Geometry check sheet. Reference: the model listing, model coordinates, mm. Give positions to 0.01 mm unless a question says otherwise; leave off trailing zeros. Write item = value, one per line. Start each with the question number.
1. Depth check by flat-ended pin: P1, Ø4, axis at x = 111.9, z = -118.65, coming from the -Y side. Enter the tip coordinate at first touch or a pass-through.
2. Thickness scan on line 1 along Z through (x, y) = (194.45, 2.4); line 2 along X through (y, z) = (0.55, -153); line 3 along X through (y, z) = (3.5, -16). Record the ranges inside material, lowest first.
3. Mould release check, pull along X, two halves, no side actions. Record for faces 1 (the flat face through (148, 3, 0)), 2 (the flat face through (300, 3, -99)), 3 (the cylindrical face through (146.173, 3.042, -119.501)): pulls with the +X half, pulls with the -X half, needs draft (parallel to the pull), parting line crosses it, or undercut.
```python
from build123d import *

# Parameters (mm, degrees)
SKETCH1_W           = 300
SKETCH1_H           = 200
BOSS_EXTRUDE1_DEPTH = 6
SKETCH6_R           = 4
CUT_EXTRUDE2_DEPTH  = 361.605047108
FILLET1_R           = 6.35
SKETCH2_R           = 1.5
CUT_EXTRUDE1_DEPTH  = 361.605047108
SKETCH13_R          = 1.6
M3_THROUGH2_DEPTH   = 364.853871767
SKETCH16_R          = 2.65
M5_THROUGH_DEPTH    = 358.420816406
SKETCH9_R           = 1.5
CUT_EXTRUDE3_DEPTH  = 361.605047108
SKETCH10_R          = 1.5
CUT_EXTRUDE5_DEPTH  = 361.605047108
SKETCH17_R          = 1.6
M3_THROUGH_DEPTH    = 361.605047108
MOVE_FACE2_BY       = 0.08
MOVE_FACE2_2_BY     = 0.08
MOVE_FACE2_3_BY     = 0.08
MOVE_FACE2_4_BY     = 0.08
MOVE_FACE2_5_BY     = 0.08
MOVE_FACE2_6_BY     = 0.08
MOVE_FACE2_7_BY     = 0.08
MOVE_FACE2_8_BY     = 0.08
MOVE_FACE2_9_BY     = 0.08
MOVE_FACE2_10_BY    = 0.08
MOVE_FACE2_11_BY    = 0.08
MOVE_FACE2_12_BY    = 0.08
MOVE_FACE2_13_BY    = 0.08
MOVE_FACE2_14_BY    = 0.08
MOVE_FACE2_15_BY    = 0.08
MOVE_FACE2_16_BY    = 0.08
MOVE_FACE2_17_BY    = 0.08
MOVE_FACE2_18_BY    = 0.08
MOVE_FACE2_19_BY    = 0.08
MOVE_FACE2_20_BY    = 0.08
MOVE_FACE2_21_BY    = 0.08
MOVE_FACE2_22_BY    = 0.08
MOVE_FACE2_23_BY    = 0.08
MOVE_FACE2_24_BY    = 0.08
MOVE_FACE2_25_BY    = 0.08
MOVE_FACE2_26_BY    = 0.08
MOVE_FACE2_27_BY    = 0.08
MOVE_FACE2_28_BY    = 0.08
MOVE_FACE2_29_BY    = 0.08
MOVE_FACE2_30_BY    = 0.08
MOVE_FACE2_31_BY    = 0.08
MOVE_FACE2_32_BY    = 0.08
MOVE_FACE2_33_BY    = 0.08
MOVE_FACE2_34_BY    = 0.08
MOVE_FACE2_35_BY    = 0.08
MOVE_FACE2_36_BY    = 0.08
MOVE_FACE2_37_BY    = 0.08
MOVE_FACE2_38_BY    = 0.08
MOVE_FACE2_39_BY    = 0.08
MOVE_FACE2_40_BY    = 0.08


with BuildPart() as part:
    # Sketch1 → Boss-Extrude1 (new body)
    with BuildSketch(Plane(origin=(0, 0, 0), x_dir=(1, 0, 0), z_dir=(0, 1, 0))):
        with Locations((150, 100)):
            Rectangle(SKETCH1_W, SKETCH1_H)
    extrude(amount=BOSS_EXTRUDE1_DEPTH)

    # Sketch6 → Cut-Extrude2 (cut, through all)
    with BuildSketch(Plane(origin=(0, 6, 0), x_dir=(1, 0, 0), z_dir=(0, 1, 0))):
        with Locations(Location((150, 118.65102, 0), (0, 0, 270))):
            Circle(SKETCH6_R)
    extrude(amount=-CUT_EXTRUDE2_DEPTH, mode=Mode.SUBTRACT)

    # Fillet1
    fillet1_edges = [part.edges().sort_by_distance(p)[0] for p in [
        (0, 3, -200),
        (300, 3, -200),
        (300, 3, 0),
        (0, 3, 0),
    ]]
    fillet(fillet1_edges, radius=FILLET1_R)

    # Sketch2 → Cut-Extrude1 (cut, through all)
    with BuildSketch(Plane(origin=(0, 6, 0), x_dir=(1, 0, 0), z_dir=(0, 1, 0))):
        with Locations(Location((6.35, 174.6, 0), (0, 0, 270))):
            Circle(SKETCH2_R)
        with Locations(Location((6.35, 49.9999, 0), (0, 0, 270))):
            Circle(SKETCH2_R)
        with Locations(Location((293.65, 49.9999, 0), (0, 0, 270))):
            Circle(SKETCH2_R)
        with Locations(Location((293.65, 174.6, 0), (0, 0, 270))):
            Circle(SKETCH2_R)
    extrude(amount=-CUT_EXTRUDE1_DEPTH, mode=Mode.SUBTRACT)

    # Sketch13 → M3-through2 (cut, through all)
    with BuildSketch(Plane(origin=(0, 6, 5.8), x_dir=(1, 0, 0), z_dir=(0, 1, 0))):
        with Locations(Location((6.35, 199.45, 0), (0, 0, 270))):
            Circle(SKETCH13_R)
        with Locations(Location((78.175, 199.45, 0), (0, 0, 270))):
            Circle(SKETCH13_R)
        with Locations(Location((221.825, 199.45, 0), (0, 0, 270))):
            Circle(SKETCH13_R)
        with Locations(Location((293.65, 199.45, 0), (0, 0, 270))):
            Circle(SKETCH13_R)
        with Locations(Location((293.65, 99.4498, 0), (0, 0, 270))):
            Circle(SKETCH13_R)
        with Locations(Location((293.65, 12.15, 0), (0, 0, 270))):
            Circle(SKETCH13_R)
        with Locations(Location((217.45, 12.15, 0), (0, 0, 270))):
            Circle(SKETCH13_R)
        with Locations(Location((82.55, 12.15, 0), (0, 0, 270))):
            Circle(SKETCH13_R)
        with Locations(Location((6.35, 12.15, 0), (0, 0, 270))):
            Circle(SKETCH13_R)
        with Locations(Location((6.35, 99.4498, 0), (0, 0, 270))):
            Circle(SKETCH13_R)
    extrude(amount=-M3_THROUGH2_DEPTH, mode=Mode.SUBTRACT)

    # Sketch16 → M5_through (cut, through all)
    with BuildSketch(Plane(origin=(0, 6, -5.8), x_dir=(1, 0, 0), z_dir=(0, -1, 0))):
        with Locations(Location((118.25, -18.65102, 0), (0, 0, 270))):
            Circle(SKETCH16_R)
        with Locations(Location((118.25, -0.55098, 0), (0, 0, 270))):
            Circle(SKETCH16_R)
        with Locations(Location((139.416666667, -0.55098, 0), (0, 0, 270))):
            Circle(SKETCH16_R)
        with Locations(Location((160.583333333, -0.55098, 0), (0, 0, 270))):
            Circle(SKETCH16_R)
        with Locations(Location((181.75, -0.55098, 0), (0, 0, 270))):
            Circle(SKETCH16_R)
        with Locations(Location((181.75, -18.65102, 0), (0, 0, 270))):
            Circle(SKETCH16_R)
    extrude(amount=M5_THROUGH_DEPTH, mode=Mode.SUBTRACT)

    # Sketch9 → Cut-Extrude3 (cut, through all)
    with BuildSketch(Plane(origin=(0, 6, 0), x_dir=(-1, 0, 0), z_dir=(0, 1, 0))):
        with Locations(Location((-118.25, -15.401, 0), (0, 0, 90))):
            Circle(SKETCH9_R)
        with Locations(Location((-150, -6.35098, 0), (0, 0, 90))):
            Circle(SKETCH9_R)
        with Locations(Location((-181.75, -15.401, 0), (0, 0, 90))):
            Circle(SKETCH9_R)
    extrude(amount=-CUT_EXTRUDE3_DEPTH, mode=Mode.SUBTRACT)

    # Sketch10 → Cut-Extrude5 (cut, through all)
    with BuildSketch(Plane(origin=(0, 6, 0), x_dir=(1, 0, 0), z_dir=(0, 1, 0))):
        with Locations(Location((150, 156.75102, 0), (0, 0, 270))):
            Circle(SKETCH10_R)
        with Locations(Location((182.995567884, 137.70102, 0), (0, 0, 270))):
            Circle(SKETCH10_R)
        with Locations(Location((182.995567884, 99.60102, 0), (0, 0, 270))):
            Circle(SKETCH10_R)
        with Locations(Location((150, 80.55102, 0), (0, 0, 270))):
            Circle(SKETCH10_R)
        with Locations(Location((117.004432116, 99.60102, 0), (0, 0, 270))):
            Circle(SKETCH10_R)
        with Locations(Location((117.004432116, 137.70102, 0), (0, 0, 270))):
            Circle(SKETCH10_R)
        with Locations(Location((105.55, 30.80102, 0), (0, 0, 270))):
            Circle(SKETCH10_R)
        with Locations(Location((105.55, 6.35, 0), (0, 0, 270))):
            Circle(SKETCH10_R)
        with Locations(Location((194.45, 6.35, 0), (0, 0, 90))):
            Circle(SKETCH10_R)
        with Locations(Location((194.45, 30.80102, 0), (0, 0, 90))):
            Circle(SKETCH10_R)
    extrude(amount=-CUT_EXTRUDE5_DEPTH, mode=Mode.SUBTRACT)

    # Sketch17 → M3-through (cut, through all)
    with BuildSketch(Plane(origin=(0, 6, 0), x_dir=(1, 0, 0), z_dir=(0, 1, 0))):
        with Locations(Location((188.1, 118.65102, 0), (0, 0, 270))):
            Circle(SKETCH17_R)
        with Locations(Location((169.05, 85.655452116, 0), (0, 0, 270))):
            Circle(SKETCH17_R)
        with Locations(Location((130.95, 85.655452116, 0), (0, 0, 270))):
            Circle(SKETCH17_R)
        with Locations(Location((111.9, 118.65102, 0), (0, 0, 270))):
            Circle(SKETCH17_R)
        with Locations(Location((130.95, 151.646587884, 0), (0, 0, 270))):
            Circle(SKETCH17_R)
        with Locations(Location((169.05, 151.646587884, 0), (0, 0, 270))):
            Circle(SKETCH17_R)
    extrude(amount=-M3_THROUGH_DEPTH, mode=Mode.SUBTRACT)

    # Move Face2: a curved face moved outward by 0.08
    add(Solid.thicken(part.faces().sort_by_distance((150, 3, -122.65102))[0], MOVE_FACE2_BY))

    # Move Face2 2: a curved face moved outward by 0.08
    add(Solid.thicken(part.faces().sort_by_distance((6.35, 3, -176.1))[0], MOVE_FACE2_2_BY))

    # Move Face2 3: a curved face moved outward by 0.08
    add(Solid.thicken(part.faces().sort_by_distance((6.35, 3, -51.4999))[0], MOVE_FACE2_3_BY))

    # Move Face2 4: a curved face moved outward by 0.08
    add(Solid.thicken(part.faces().sort_by_distance((293.65, 3, -51.4999))[0], MOVE_FACE2_4_BY))

    # Move Face2 5: a curved face moved outward by 0.08
    add(Solid.thicken(part.faces().sort_by_distance((293.65, 3, -176.1))[0], MOVE_FACE2_5_BY))

    # Move Face2 6: a curved face moved outward by 0.08
    add(Solid.thicken(part.faces().sort_by_distance((6.35, 3, -195.25))[0], MOVE_FACE2_6_BY))

    # Move Face2 7: a curved face moved outward by 0.08
    add(Solid.thicken(part.faces().sort_by_distance((78.175, 3, -195.25))[0], MOVE_FACE2_7_BY))

    # Move Face2 8: a curved face moved outward by 0.08
    add(Solid.thicken(part.faces().sort_by_distance((221.825, 3, -195.25))[0], MOVE_FACE2_8_BY))

    # Move Face2 9: a curved face moved outward by 0.08
    add(Solid.thicken(part.faces().sort_by_distance((293.65, 3, -195.25))[0], MOVE_FACE2_9_BY))

    # Move Face2 10: a curved face moved outward by 0.08
    add(Solid.thicken(part.faces().sort_by_distance((293.65, 3, -95.2498))[0], MOVE_FACE2_10_BY))

    # Move Face2 11: a curved face moved outward by 0.08
    add(Solid.thicken(part.faces().sort_by_distance((293.65, 3, -7.95))[0], MOVE_FACE2_11_BY))

    # Move Face2 12: a curved face moved outward by 0.08
    add(Solid.thicken(part.faces().sort_by_distance((217.45, 3, -7.95))[0], MOVE_FACE2_12_BY))

    # Move Face2 13: a curved face moved outward by 0.08
    add(Solid.thicken(part.faces().sort_by_distance((82.55, 3, -7.95))[0], MOVE_FACE2_13_BY))

    # Move Face2 14: a curved face moved outward by 0.08
    add(Solid.thicken(part.faces().sort_by_distance((6.35, 3, -7.95))[0], MOVE_FACE2_14_BY))

    # Move Face2 15: a curved face moved outward by 0.08
    add(Solid.thicken(part.faces().sort_by_distance((6.35, 3, -95.2498))[0], MOVE_FACE2_15_BY))

    # Move Face2 16: a curved face moved outward by 0.08
    add(Solid.thicken(part.faces().sort_by_distance((118.25, 3, -21.80102))[0], MOVE_FACE2_16_BY))

    # Move Face2 17: a curved face moved outward by 0.08
    add(Solid.thicken(part.faces().sort_by_distance((118.25, 3, -3.70098))[0], MOVE_FACE2_17_BY))

    # Move Face2 18: a curved face moved outward by 0.08
    add(Solid.thicken(part.faces().sort_by_distance((139.416666667, 3, -3.70098))[0], MOVE_FACE2_18_BY))

    # Move Face2 19: a curved face moved outward by 0.08
    add(Solid.thicken(part.faces().sort_by_distance((160.583333333, 3, -3.70098))[0], MOVE_FACE2_19_BY))

    # Move Face2 20: a curved face moved outward by 0.08
    add(Solid.thicken(part.faces().sort_by_distance((181.75, 3, -3.70098))[0], MOVE_FACE2_20_BY))

    # Move Face2 21: a curved face moved outward by 0.08
    add(Solid.thicken(part.faces().sort_by_distance((181.75, 3, -21.80102))[0], MOVE_FACE2_21_BY))

    # Move Face2 22: a curved face moved outward by 0.08
    add(Solid.thicken(part.faces().sort_by_distance((118.25, 3, -16.901))[0], MOVE_FACE2_22_BY))

    # Move Face2 23: a curved face moved outward by 0.08
    add(Solid.thicken(part.faces().sort_by_distance((150, 3, -7.85098))[0], MOVE_FACE2_23_BY))

    # Move Face2 24: a curved face moved outward by 0.08
    add(Solid.thicken(part.faces().sort_by_distance((181.75, 3, -16.901))[0], MOVE_FACE2_24_BY))

    # Move Face2 25: a curved face moved outward by 0.08
    add(Solid.thicken(part.faces().sort_by_distance((150, 3, -158.25102))[0], MOVE_FACE2_25_BY))

    # Move Face2 26: a curved face moved outward by 0.08
    add(Solid.thicken(part.faces().sort_by_distance((182.995567884, 3, -139.20102))[0], MOVE_FACE2_26_BY))

    # Move Face2 27: a curved face moved outward by 0.08
    add(Solid.thicken(part.faces().sort_by_distance((182.995567884, 3, -101.10102))[0], MOVE_FACE2_27_BY))

    # Move Face2 28: a curved face moved outward by 0.08
    add(Solid.thicken(part.faces().sort_by_distance((150, 3, -82.05102))[0], MOVE_FACE2_28_BY))

    # Move Face2 29: a curved face moved outward by 0.08
    add(Solid.thicken(part.faces().sort_by_distance((117.004432116, 3, -101.10102))[0], MOVE_FACE2_29_BY))

    # Move Face2 30: a curved face moved outward by 0.08
    add(Solid.thicken(part.faces().sort_by_distance((117.004432116, 3, -139.20102))[0], MOVE_FACE2_30_BY))

    # Move Face2 31: a curved face moved outward by 0.08
    add(Solid.thicken(part.faces().sort_by_distance((105.55, 3, -32.30102))[0], MOVE_FACE2_31_BY))

    # Move Face2 32: a curved face moved outward by 0.08
    add(Solid.thicken(part.faces().sort_by_distance((105.55, 3, -7.85))[0], MOVE_FACE2_32_BY))

    # Move Face2 33: a curved face moved outward by 0.08
    add(Solid.thicken(part.faces().sort_by_distance((194.45, 3, -4.85))[0], MOVE_FACE2_33_BY))

    # Move Face2 34: a curved face moved outward by 0.08
    add(Solid.thicken(part.faces().sort_by_distance((194.45, 3, -29.30102))[0], MOVE_FACE2_34_BY))

    # Move Face2 35: a curved face moved outward by 0.08
    add(Solid.thicken(part.faces().sort_by_distance((188.1, 3, -120.25102))[0], MOVE_FACE2_35_BY))

    # Move Face2 36: a curved face moved outward by 0.08
    add(Solid.thicken(part.faces().sort_by_distance((169.05, 3, -87.255452116))[0], MOVE_FACE2_36_BY))

    # Move Face2 37: a curved face moved outward by 0.08
    add(Solid.thicken(part.faces().sort_by_distance((130.95, 3, -87.255452116))[0], MOVE_FACE2_37_BY))

    # Move Face2 38: a curved face moved outward by 0.08
    add(Solid.thicken(part.faces().sort_by_distance((111.9, 3, -120.25102))[0], MOVE_FACE2_38_BY))

    # Move Face2 39: a curved face moved outward by 0.08
    add(Solid.thicken(part.faces().sort_by_distance((130.95, 3, -153.246587884))[0], MOVE_FACE2_39_BY))

    # Move Face2 40: a curved face moved outward by 0.08
    add(Solid.thicken(part.faces().sort_by_distance((169.05, 3, -153.246587884))[0], MOVE_FACE2_40_BY))


solid = part.part
```
Answers:
q1.P1 = 0
q2.line_1 = -200 to -32.22, -29.38 to -7.77, -4.93 to 0
q2.line_2 = 0 to 130.26, 131.64 to 168.36, 169.74 to 300
q2.line_3 = 0 to 116.96, 119.54 to 180.46, 183.04 to 300
q3.face_1 = needs draft
q3.face_2 = pulls with the +X half
q3.face_3 = undercut
